```python
from build123d import *

# Parameters (mm, degrees)
F0_W     = 34
F0_H     = 35
F1_DEPTH = 8
F2_W     = 5
F2_H     = 8
F3_DEPTH = 11
F4_R     = 3.99999
F6_DEPTH = 2
F7_R     = 1
F9_DEPTH = 2
F10_R    = 1
F11_R    = 0.5


# Not quite as in the source:
# - a fillet or chamfer is up to 0.001 mm smaller than in the source, because OpenCascade refuses the exact size


with BuildPart() as f1:
    # F0 (on Front) → F1 (new body)
    with BuildSketch(Plane.XZ):
        with Locations((17, 17.5)):
            Rectangle(F0_W, F0_H)
    extrude(amount=-F1_DEPTH)

    # F2 (on face) → F3 (join)
    with BuildSketch(Plane(origin=(0, 0, 0), x_dir=(1, 0, 0), z_dir=(0, 0, -1))):
        with Locations((31.5, -4)):
            Rectangle(F2_W, F2_H)
        with Locations((2.5, -4)):
            Rectangle(F2_W, F2_H)
    extrude(amount=F3_DEPTH)

    # F4 (radius 4 in the source; OpenCascade refuses exactly that, so slightly less here)
    f4_edges = [f1.edges().sort_by_distance(p)[0] for p in [
        (2.5, 0, -11),
        (2.5, 8, -11),
        (31.5, 8, -11),
        (31.5, 0, -11),
    ]]
    fillet(f4_edges, radius=F4_R)

    # F5 (on face) → F6 (join)
    with BuildSketch(Plane(origin=(29, 0, 0), x_dir=(0, -1, 0), z_dir=(-1, 0, 0))):
        with BuildLine():
            Line((-5.027864045, -7), (-2.027864045, -7))
            ThreePointArc((-2.027864045, -7), (-3.527864045, -5.5), (-5.027864045, -7))
        make_face()
        with BuildLine():
            ThreePointArc((-5.027864045, -7), (-3.527864045, -8.5), (-2.027864045, -7))
            Line((-2.027864045, -7), (-5.027864045, -7))
        make_face()
    extrude(amount=F6_DEPTH)

    # F7
    f7_edges = [f1.edges().sort_by_distance(p)[0] for p in [
        (27, 2.027864, -7),
    ]]
    fillet(f7_edges, radius=F7_R)

    # F8 (on face) → F9 (join)
    with BuildSketch(Plane.YZ.offset(5)):
        with BuildLine():
            Line((2.5, -7), (5.5, -7))
            ThreePointArc((5.5, -7), (4, -5.5), (2.5, -7))
        make_face()
        with BuildLine():
            ThreePointArc((2.5, -7), (4, -8.5), (5.5, -7))
            Line((5.5, -7), (2.5, -7))
        make_face()
    extrude(amount=F9_DEPTH)

    # F10
    f10_edges = [f1.edges().sort_by_distance(p)[0] for p in [
        (7, 5.5, -7),
    ]]
    fillet(f10_edges, radius=F10_R)

    # F11
    f11_edges = [f1.edges().sort_by_distance(p)[0] for p in [
        (0, 0, 13.999995),
        (2.5, 0, -7.00001),
        (17, 0, 35),
        (5, 0, -3.500005),
        (34, 0, 13.999995),
        (17, 0, 0),
        (31.5, 0, -7.00001),
        (29, 0, -3.500005),
        (0, 8, 13.999995),
        (2.5, 8, -7.00001),
        (17, 8, 35),
        (5, 8, -3.500005),
        (34, 8, 13.999995),
        (17, 8, 0),
        (31.5, 8, -7.00001),
        (29, 8, -3.500005),
        (34, 4, 35),
        (0, 4, 35),
    ]]
    fillet(f11_edges, radius=F11_R)


solid = f1.part
```
Can you work these out from the model? Positions are in its coordinate system, mm. A direction names the side the tool comes from. Give positions to 0.01 mm unless a question says otherwise; leave off trailing zeros. Order: outer loops, then holes, each group sorted by start corner. A loop starts at its lowest first (then second) coordinate and runs counter-clockwise, first axis right, second up. Notation, with made-up numbers: (51.5, -27.5) - (66.5, -27.5) arc R17 cw to (66.5, -17.5) - close; hole circle Ø4 at (20.5, -13.75). An arc over 180 degrees is marked (long way). Use a Markdown table: item, result. Add a question column.
Q1. I'm going to push a flat-ended pin straight in: pin 1 (1.5 mm diameter, centred on x = 3.5, y = 6.5, fed in from -Z). Where does the tip first touch, or does it pass through?
Q2. If we section it at A-A on z = -4: Write out the boundary of the cut face in (x, y).
Q3. On a 3-axis mill with a long thin cutter (end or side, diameter ignored), from which of +Z, -Z, +X, -X, +Y, -Y can I reach the whole of each face in a straight line? I mean faces 1 (the cylindrical face through (31.528, 1.203, -9.859)), 2 (the cylindrical face through (5.493, 4.325, -5.536)), 3 (the flat face through (7, 4, -7)). Say none if no direction works.
Q4. If we mould it in two halves opening along X, with no side actions, what happens to faces 4 (the flat face through (34, 4, 12)), 5 (the flat face through (17, 0, 19)), 6 (the flat face through (27, 3.5, -7))? For each: released by +X, released by -X, zero draft, split by the parting line, or undercut.
Q5. Please list where these lines run through material, in increasing order: line 1 along X through (y, z) = (6.5, -5.5); line 2 along Z through (x, y) = (30, 3.75); line 3 along Z through (x, y) = (15, 5.5).
Q6. If we section it at B-B on x = 23: Write out the boundary of the cut face in (y, z).
Answers follow:
| question | item | result |
|---|---|---|
| 1 | pin 1 | stops at z = -10.6 |
| 2 | outline | (0, 0.5) arc R0.5 ccw to (0.5, 0) - (4.5, 0) arc R0.5 ccw to (5, 0.5) - (5, 7.5) arc R0.5 ccw to (4.5, 8) - (0.5, 8) arc R0.5 ccw to (0, 7.5) - close; (29, 0.5) arc R0.5 ccw to (29.5, 0) - (33.5, 0) arc R0.5 ccw to (34, 0.5) - (34, 7.5) arc R0.5 ccw to (33.5, 8) - (29.5, 8) arc R0.5 ccw to (29, 7.5) - close |
| 3 | face 1 | -Z, +X, -X, -Y |
| 3 | face 2 | none |
| 3 | face 3 | -Z, +Y, -Y |
| 4 | face 4 | released by +X |
| 4 | face 5 | zero draft |
| 4 | face 6 | undercut |
| 5 | line 1 | x = 0 to 5, 29 to 34 |
| 5 | line 2 | z = -10.99 to 35 |
| 5 | line 3 | z = 0 to 35 |
| 6 | outline | (0, 0.5) arc R0.5 ccw to (0.5, 0) - (7.5, 0) arc R0.5 ccw to (8, 0.5) - (8, 34.5) arc R0.5 ccw to (7.5, 35) - (0.5, 35) arc R0.5 ccw to (0, 34.5) - close |
